CAD build for the part. Positions are in the model's coordinates, mm. A direction names the side the tool comes from. Coordinates: 2 decimals unless noted, no trailing zeros. Answer in a Markdown table with one row per item. Add a question column.
Q1. Pin check, flat tips, straight feed: pin 1 (8.5 mm diameter, centred on x = -69.5, y = 294.5, fed in from +Z); pin 2 (14 mm diameter, centred on x = -122, z = 25.5, fed in from +Y); pin 3 (6 mm diameter, centred on y = 111, z = 24.5, fed in from -X); pin 4 (10 mm diameter, centred on x = 253, z = 25, fed in from +Y). Stop position of each tip, or through.
Q2. Two-plate mould, pull along Y, no slides. Class faces 3 (the flat face through (-3, 288, 12.7)), 4 (the flat face through (9, 304.8, 0)), 5 (the flat face through (-9, -304.8, 0)): +Y half, -Y half, draft (parallel to the pull), parting line (faces both ways), or undercut.
Q3. Drill centre lines: line 1 along Y through (x, z) = (-597.75, 0); line 2 along Z through (x, y) = (-617, -198); line 3 along Y through (x, z) = (-508, -10). Where is each one in solid material? Low to high. Write a range as from..to.
Q4. 3-axis set-ups, long thin cutter, end or side, ignore diameter. For faces 1 (the flat face through (609.6, 4, 0)), 2 (the flat face through (-3, -288, 6.35)): which of +Z, -Z, +X, -X, +Y, -Y reach the whole face in a straight line?
```python
from build123d import *

# Parameters (mm, degrees)
CUT_EXTRUDE4_REACH  = 1221.2
SKETCH4_R           = 5.08
SKETCH5_R           = 7.62
SKETCH5_R_2         = 5.08
BOSS_EXTRUDE3_DEPTH = 25.4
SKETCH7_W           = 1219.2
SKETCH7_H           = 2.54
BOSS_EXTRUDE4_DEPTH = 12.7


with BuildPart() as part:
    # Sweep1: sweep along a path in Sketch2
    with BuildLine(Plane.XY) as sweep1_path:
        Line((609.6, -304.8), (-609.6, -304.8))
        Line((-609.6, -304.8), (-609.6, 304.8))
        Line((-609.6, 304.8), (609.6, 304.8))
        Line((609.6, 304.8), (609.6, -304.8))
    # Sketch3 → Sweep1 (sweep)
    with BuildSketch(Plane(origin=(0, 0, 0), x_dir=(0, 0, -1), z_dir=(1, 0, 0))):
        Polygon((-19.05, 304.8), (19.05, 304.8), (19.05, 285.75), (13.97, 285.75), (12.7, 287.02), (12.7, 297.18), (11.43, 298.45), (7.62, 298.45), (6.35, 297.18), (6.35, 287.02), (5.08, 285.75), (-5.08, 285.75), (-6.35, 287.02), (-6.35, 297.18), (-7.62, 298.45), (-11.43, 298.45), (-12.7, 297.18), (-12.7, 287.02), (-13.97, 285.75), (-19.05, 285.75), align=None)
    sweep(path=sweep1_path.line, transition=Transition.RIGHT)

    # Sketch4 → Cut-Extrude4 (cut, up to next)
    with BuildSketch(Plane.ZY.offset(609.6), mode=Mode.PRIVATE) as cut_extrude4_sk1:
        with Locations((0, -266.7)):
            Circle(SKETCH4_R)
    cut_extrude4_tool1 = extrude(cut_extrude4_sk1.sketch, amount=-CUT_EXTRUDE4_REACH, mode=Mode.PRIVATE) & part.part
    add(cut_extrude4_tool1.solids().sort_by_distance((-609.6, -266.7, 0))[0], mode=Mode.SUBTRACT)
    # Sketch4 → Cut-Extrude4 (cut, up to next)
    with BuildSketch(Plane.ZY.offset(609.6), mode=Mode.PRIVATE) as cut_extrude4_sk2:
        with Locations((0, -243.84)):
            Circle(SKETCH4_R)
    cut_extrude4_tool2 = extrude(cut_extrude4_sk2.sketch, amount=-CUT_EXTRUDE4_REACH, mode=Mode.PRIVATE) & part.part
    add(cut_extrude4_tool2.solids().sort_by_distance((-609.6, -243.84, 0))[0], mode=Mode.SUBTRACT)
    # Sketch4 → Cut-Extrude4 (cut, up to next)
    with BuildSketch(Plane.ZY.offset(609.6), mode=Mode.PRIVATE) as cut_extrude4_sk3:
        with Locations((0, -220.98)):
            Circle(SKETCH4_R)
    cut_extrude4_tool3 = extrude(cut_extrude4_sk3.sketch, amount=-CUT_EXTRUDE4_REACH, mode=Mode.PRIVATE) & part.part
    add(cut_extrude4_tool3.solids().sort_by_distance((-609.6, -220.98, 0))[0], mode=Mode.SUBTRACT)
    # Sketch4 → Cut-Extrude4 (cut, up to next)
    with BuildSketch(Plane.ZY.offset(609.6), mode=Mode.PRIVATE) as cut_extrude4_sk4:
        with Locations((0, -198.12)):
            Circle(SKETCH4_R)
    cut_extrude4_tool4 = extrude(cut_extrude4_sk4.sketch, amount=-CUT_EXTRUDE4_REACH, mode=Mode.PRIVATE) & part.part
    add(cut_extrude4_tool4.solids().sort_by_distance((-609.6, -198.12, 0))[0], mode=Mode.SUBTRACT)

    # Sketch5 → Boss-Extrude3 (add)
    with BuildSketch(Plane.ZY.offset(609.6)):
        with Locations((0, -198.12)):
            Circle(SKETCH5_R)
        with Locations((0, -198.12)):
            Circle(SKETCH5_R_2, mode=Mode.SUBTRACT)
        with Locations((0, -220.98)):
            Circle(SKETCH5_R)
        with Locations((0, -220.98)):
            Circle(SKETCH5_R_2, mode=Mode.SUBTRACT)
        with Locations((0, -243.84)):
            Circle(SKETCH5_R)
        with Locations((0, -243.84)):
            Circle(SKETCH5_R_2, mode=Mode.SUBTRACT)
        with Locations((0, -266.7)):
            Circle(SKETCH5_R)
        with Locations((0, -266.7)):
            Circle(SKETCH5_R_2, mode=Mode.SUBTRACT)
    extrude(amount=BOSS_EXTRUDE3_DEPTH)

    # Sketch7 → Boss-Extrude4 (add)
    with BuildSketch(Plane.XY.offset(19.05)):
        with Locations((0, 287.02)):
            Rectangle(SKETCH7_W, SKETCH7_H)
    boss_extrude4 = extrude(amount=BOSS_EXTRUDE4_DEPTH)

    # Mirror1: Boss-Extrude4 across plane
    add(boss_extrude4.mirror(Plane.ZX))


solid = part.part
```
Checked values:
| question | item | result |
|---|---|---|
| 1 | pin 1 | stops at z = 19.05 |
| 1 | pin 2 | stops at y = 304.8 |
| 1 | pin 3 | passes through |
| 1 | pin 4 | stops at y = 288.29 |
| 2 | face 3 | undercut |
| 2 | face 4 | +Y half |
| 2 | face 5 | -Y half |
| 3 | line 1 | y = -304.8..-271.78, -261.62..-248.92, -238.76..-226.06, -215.9..-203.2, -193.04..304.8 |
| 3 | line 2 | z = -7.62..-5.08, 5.08..7.62 |
| 3 | line 3 | y = -304.8..-298.45, 298.45..304.8 |
| 4 | face 1 | +Z, -Z, +X, +Y, -Y |
| 4 | face 2 | none |
